```python
from build123d import *

# Parameters (mm, degrees)
F0_W     = 35
F0_H     = 35
F0_R     = 11.285
F0_R_2   = 1
F1_DEPTH = 2
F3_DEPTH = 35
F4_DEPTH = 25


with BuildPart() as f1:
    # F0 (on Top) → F1 (new body)
    with BuildSketch(Plane.XY):
        Rectangle(F0_W, F0_H)
        Circle(F0_R, mode=Mode.SUBTRACT)
        Circle(F0_R)
        with Locations((0, -8.785)):
            Circle(F0_R_2, mode=Mode.SUBTRACT)
        with Locations((-7.6080331722, 4.3925)):
            Circle(F0_R_2, mode=Mode.SUBTRACT)
        with Locations((7.6080331722, 4.3925)):
            Circle(F0_R_2, mode=Mode.SUBTRACT)
    extrude(amount=F1_DEPTH)

    # F2 (on face) → F3 (join, through all)
    with BuildSketch(Plane.XZ.offset(17.5)):
        Polygon((17.5, -5.9556164779), (17.5, 0), (-17.5, 0), align=None)
    extrude(amount=-F3_DEPTH)

    # F4 (cut): faces of the model
    f4_faces = [f1.faces().sort_by_distance(p)[0] for p in [
        (7.6080331722, 4.3925, 0),
        (0, -8.785, 0),
        (-7.6080331722, 4.3925, 0),
    ]]
    extrude(f4_faces, amount=-F4_DEPTH, mode=Mode.SUBTRACT)


solid = f1.part
```
Check sheet for the modelled part. Datum: model origin and axes. Units: mm. Give positions to 0.01 mm unless a question says otherwise; leave off trailing zeros. Order: outer loops, then holes, each group sorted by start corner. A loop starts at its lowest first (then second) coordinate and runs counter-clockwise, first axis right, second up. Notation, with made-up numbers: (4, 24.25) -> (62, 24.25) arc R19 cw to (62, 61.25) -> close; hole circle Ø4 at (39.25, 54). An arc over 180 degrees is marked (long way). Return JSON: item names as keys, results as strings.
1. Cross-section at D-D, the plane x = 3.5. Record the cut outline in (y, z).
From the geometry:
{"outline": "(-17.5, -3.57) -> (17.5, -3.57) -> (17.5, 2) -> (-17.5, 2) -> close"}
2. Cross-section at B-B, the plane z = -1. Record the cut outline in (x, y) (1 decimal), plus the area to 3 significant figures.
From the geometry:
{"outline": "(-11.6, -17.5) -> (17.5, -17.5) -> (17.5, 17.5) -> (-11.6, 17.5) -> close; hole circle Ø2 at (-7.6, 4.4); hole circle Ø2 at (0, -8.8); hole circle Ø2 at (7.6, 4.4)", "area": "1,010 mm^2"}
3. Cross-section at C-C, the plane y = -5.5. Record the cut outline in (x, z), plus the area to 3 significant figures.
From the geometry:
{"outline": "(-17.5, 0) -> (17.5, -5.96) -> (17.5, 2) -> (-17.5, 2) -> close", "area": "174 mm^2"}
4. Material ranges on probe 1 along Z at (x, y) = (1, -2); probe 2 along Y at (x, z) = (-7, 1.5); probe 3 along Z at (x, y) = (6, 13), recorded low to high. Write a range as [from, to].
From the geometry:
{"probe 1": "[-3.15, 2]", "probe 2": "[-17.5, 3.6], [5.19, 17.5]", "probe 3": "[-4, 2]"}
5. Go/stop test with flat-tipped pins: P1, Ø1.6, axis at x = 0, y = -8.785, coming from the +Z side; P2, Ø6, axis at x = 5, y = 10.5, coming from the -Z side. Record where each tip stops, or that it passes through.
From the geometry:
{"P1": "through", "P2": "z = -4.34"}
6. Cross-section at A-A, the plane x = 0. Record the cut outline in (y, z) (3 decimals), plus the area to 3 significant figures.
From the geometry:
{"outline": "(-17.5, -2.978) -> (-9.785, -2.978) -> (-9.785, 2) -> (-17.5, 2) -> close; (-7.785, -2.978) -> (17.5, -2.978) -> (17.5, 2) -> (-7.785, 2) -> close", "area": "164 mm^2"}
